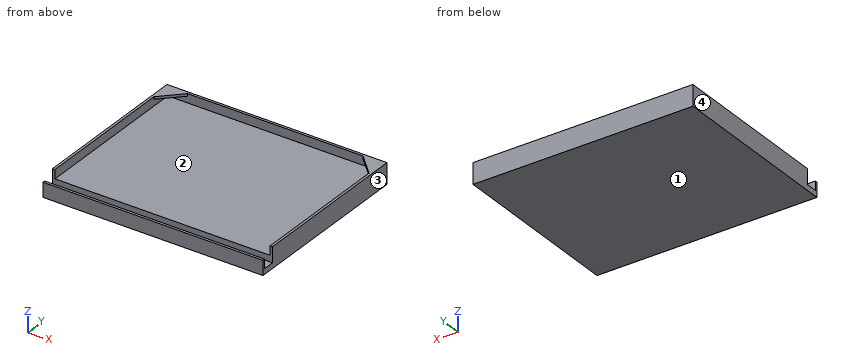
from build123d import *

# Parameters (mm, degrees)
SKETCH1_W            = 281.94
SKETCH1_H            = 228.6
BOSS_EXTRUDE2_DEPTH  = 25.4
SKETCH3_W            = 281.94
SKETCH3_H            = 17.526
CUT_EXTRUDE1_DEPTH   = 8.128
SKETCH4_W            = 11.43
SKETCH4_H            = 211.074
BOSS_EXTRUDE4_DEPTH  = 3.175
SKETCH5_W            = 278.765
SKETCH5_H            = 11.43
BOSS_EXTRUDE9_DEPTH  = 3.175
SKETCH9_W            = 11.43
SKETCH9_H            = 207.899
BOSS_EXTRUDE10_DEPTH = 3.175
SKETCH8_W            = 281.94
SKETCH8_H            = 11.43
BOSS_EXTRUDE11_DEPTH = 3.175
SKETCH10_W           = 281.94
SKETCH10_H           = 14.351
CUT_EXTRUDE2_DEPTH   = 10.16
SKETCH11_W           = 275.59
SKETCH11_H           = 207.899
CUT_EXTRUDE3_DEPTH   = 10.16
CUT_EXTRUDE4_DEPTH   = 10.16
SKETCH13_W           = 281.94
SKETCH13_H           = 3.175
CUT_EXTRUDE5_DEPTH   = 10.16
SHELL4_START         = -65.823170732
SHELL4_DEPTH         = 276.86
BOSS_EXTRUDE12_DEPTH = 3.175


# Read off the part's stored shape, not the designer's step: Shell4
with BuildPart() as part:
    # Sketch1 → Boss-Extrude2 (new body)
    with BuildSketch(Plane.XY):
        with Locations((72.606829268, 16.339634146)):
            Rectangle(SKETCH1_W, SKETCH1_H)
    extrude(amount=BOSS_EXTRUDE2_DEPTH)

    # Sketch3 → Cut-Extrude1 (cut)
    with BuildSketch(Plane.XY.offset(25.4)):
        with Locations((72.606829268, -89.197365854)):
            Rectangle(SKETCH3_W, SKETCH3_H)
    extrude(amount=-CUT_EXTRUDE1_DEPTH, mode=Mode.SUBTRACT)



with BuildPart() as body_2:
    # Sketch4 → Boss-Extrude4 (new body)
    with BuildSketch(Plane.ZY.offset(68.363170732)):
        with Locations((31.115, 25.102634146)):
            Rectangle(SKETCH4_W, SKETCH4_H)
    extrude(amount=-BOSS_EXTRUDE4_DEPTH)


with BuildPart() as part_1:
    add(part.part)

    add(body_2.part)  # Boss-Extrude9 merges body 2
    # Sketch5 → Boss-Extrude9 (add)
    with BuildSketch(Plane(origin=(0, 130.639634146, 0), x_dir=(1, 0, 0), z_dir=(0, 1, 0))):
        with Locations((74.194329268, -31.115)):
            Rectangle(SKETCH5_W, SKETCH5_H)
    extrude(amount=-BOSS_EXTRUDE9_DEPTH)

    # Sketch9 → Boss-Extrude10 (add)
    with BuildSketch(Plane(origin=(213.576829268, 0, 0), x_dir=(0, 0, -1), z_dir=(1, 0, 0))):
        with Locations((-31.115, 23.515134146)):
            Rectangle(SKETCH9_W, SKETCH9_H)
    extrude(amount=-BOSS_EXTRUDE10_DEPTH)


with BuildPart() as body_2_2:
    # Sketch8 → Boss-Extrude11 (new body)
    with BuildSketch(Plane.XZ.offset(97.960365854)):
        with Locations((72.606829268, 22.987)):
            Rectangle(SKETCH8_W, SKETCH8_H)
    extrude(amount=-BOSS_EXTRUDE11_DEPTH)

    # Combine1: union part
    add(part_1.part)

    # Sketch10 → Cut-Extrude2 (cut)
    with BuildSketch(Plane.XY.offset(17.272)):
        with Locations((72.606829268, -87.609865854)):
            Rectangle(SKETCH10_W, SKETCH10_H)
    extrude(amount=-CUT_EXTRUDE2_DEPTH, mode=Mode.SUBTRACT)

    # Sketch11 → Cut-Extrude3 (cut)
    with BuildSketch(Plane.XY.offset(25.4)):
        with Locations((72.606829268, 23.515134146)):
            Rectangle(SKETCH11_W, SKETCH11_H)
    extrude(amount=-CUT_EXTRUDE3_DEPTH, mode=Mode.SUBTRACT)

    # Sketch12 → Cut-Extrude4 (cut)
    with BuildSketch(Plane.XY.offset(36.83)):
        Polygon((-68.363170732, -80.434365854), (-65.188170732, -80.434365854), (-65.188170732, 127.464634146), (210.401829268, 127.464634146), (210.401829268, -80.434365854), (213.576829268, -80.434365854), (213.576829268, 130.639634146), (-68.363170732, 130.639634146), align=None)
    extrude(amount=-CUT_EXTRUDE4_DEPTH, mode=Mode.SUBTRACT)

    # Sketch13 → Cut-Extrude5 (cut)
    with BuildSketch(Plane.XY.offset(28.702)):
        with Locations((72.606829268, -96.372865854)):
            Rectangle(SKETCH13_W, SKETCH13_H)
    extrude(amount=-CUT_EXTRUDE5_DEPTH, mode=Mode.SUBTRACT)

    # Shell4 outline → Shell4 (cut)
    with BuildSketch(Plane.YZ.offset(SHELL4_START)):
        Polygon((-95.420365854, 4.572), (-95.420365854, 2.54), (128.099634146, 2.54), (128.099634146, 12.7), (-77.894365854, 12.7), (-77.894365854, 4.572), align=None)
    extrude(amount=SHELL4_DEPTH, mode=Mode.SUBTRACT)

    # Sketch14 → Boss-Extrude12 (add)
    with BuildSketch(Plane.XY.offset(26.67)):
        Polygon((-65.188170732, 102.064634146), (-39.788170732, 127.464634146), (-65.188170732, 127.464634146), align=None)
        Polygon((185.001829268, 127.464634146), (210.401829268, 102.064634146), (210.401829268, 127.464634146), align=None)
    extrude(amount=-BOSS_EXTRUDE12_DEPTH)


solid = body_2_2.part
For this review, take the finished solid that the model builds, in its own axes (mm). Face numbers are marked on the shaded views. Round coordinates to 2 decimals unless told otherwise and drop trailing zeros. Loops run counter-clockwise (first coordinate to the right, second up) from the corner with the lowest first, then second, coordinate; pieces in that order, holes last. Notation, with made-up numbers: (-32, -16) - (-4, -16) arc R18 ccw to (-4, -11) - close; hole circle Ø7 at (-32.5, 7). An arc over 180 degrees is marked (long way). One line per item, written item: value. Start each with the question number.
Item 1: For L1, parallel to Y at x = -15.5, z = 8.25; L2, parallel to Z at x = 41, y = 10.5; L3, parallel to X at y = 35, z = 19.25, list the stretches that pass through material, from the lowest coordinate up.
Item 2: Clearance check with flat-ended pins moving along their axes: pin 1 Ø1.5 at (x, y) = (152, 103) entering from -Z; pin 2 Ø12 at (x, y) = (129, -15) entering from +Z; pin 3 Ø2.5 at (x, y) = (98.5, -96) entering from +Z. State where each tip first meets the part, or that it passes through.
Item 3: Take a section at A-A (x = -1.5). Give the boundary of the cut face in (y, z).
Item 4: Take a section at B-B (y = 93). Give the boundary of the cut face in (x, z), plus the area to 3 significant figures.
Item 5: The part is to be moulded in two halves that separate along X. For the marked faces 1, 2, 3 and 4, say which applies: +X half, -X half, draft (parallel to the pull), parting line (faces both ways), or undercut.
Answer below:
1. L1: y = -97.96 to -94.79, -80.43 to -77.89, 128.1 to 130.64
1. L2: z = 0 to 2.54, 12.7 to 15.24
1. L3: x = -68.36 to -65.19, 210.4 to 213.58
2. pin 1: stops at z = 0
2. pin 2: stops at z = 15.24
2. pin 3: stops at z = 18.54
3. outline: (-97.96, 0) - (130.64, 0) - (130.64, 26.67) - (127.46, 26.67) - (127.46, 15.24) - (-80.43, 15.24) - (-80.43, 7.11) - (-94.79, 7.11) - (-94.79, 18.54) - (-97.96, 18.54) - close; hole (-95.42, 2.54) - (128.1, 2.54) - (128.1, 12.7) - (-77.89, 12.7) - (-77.89, 4.57) - (-95.42, 4.57) - close
4. outline: (-68.36, 0) - (213.58, 0) - (213.58, 26.67) - (210.4, 26.67) - (210.4, 15.24) - (-65.19, 15.24) - (-65.19, 26.67) - (-68.36, 26.67) - close; hole (-65.82, 2.54) - (211.04, 2.54) - (211.04, 12.7) - (-65.82, 12.7) - close
4. area: 1,560 mm2
5. face 1: draft
5. face 2: undercut
5. face 3: +X half
5. face 4: -X half
